Part model, mm, in its own coordinate system. Give positions to 0.01 mm unless a question says otherwise; leave off trailing zeros. Write each loop counter-clockwise with the first axis right and the second up, starting at its lowest first coordinate (ties: lowest second). Pieces come first, ordered by that corner, then holes.
```python
from build123d import *

# Parameters (mm, degrees)
SKETCH1_W               = 279.4
SKETCH1_H               = 90.8685
BOSS_EXTRUDE1_DEPTH     = 2.54
SKETCH2_W               = 12.7
SKETCH2_H               = 2.54
CUT_EXTRUDE1_DEPTH      = 147.92451352
LPATTERN1_COUNT         = 3
LPATTERN1_PITCH         = 25.4
MIRROR1_COPY_1_SKETCH_W = 12.7
MIRROR1_COPY_1_SKETCH_H = 2.54
MIRROR1_COPY_1_DEPTH    = 147.92451352
MIRROR1_COPY_2_SKETCH_W = 12.7
MIRROR1_COPY_2_SKETCH_H = 2.54
MIRROR1_COPY_2_DEPTH    = 147.92451352
SKETCH3_W               = 2.54
SKETCH3_H               = 25.4
CUT_EXTRUDE2_DEPTH      = 147.92451352
LPATTERN2_COUNT         = 2
LPATTERN2_PITCH         = 50.8
MIRROR2_COPY_1_SKETCH_W = 2.54
MIRROR2_COPY_1_SKETCH_H = 25.4
MIRROR2_COPY_1_DEPTH    = 147.92451352
SKETCH4_W               = 2.54
SKETCH4_H               = 12.7
CUT_EXTRUDE3_DEPTH      = 147.92451352
LPATTERN3_COUNT         = 3
LPATTERN3_PITCH         = 25.4
MIRROR3_COPY_1_SKETCH_W = 2.54
MIRROR3_COPY_1_SKETCH_H = 12.7
MIRROR3_COPY_1_DEPTH    = 147.92451352
MIRROR3_COPY_2_SKETCH_W = 2.54
MIRROR3_COPY_2_SKETCH_H = 12.7
MIRROR3_COPY_2_DEPTH    = 147.92451352
SKETCH5_W               = 25.4
SKETCH5_H               = 2.54
SKETCH5_W_2             = 10.76325
CUT_EXTRUDE4_DEPTH      = 147.92451352


with BuildPart() as part:
    # Sketch1 → Boss-Extrude1 (new body)
    with BuildSketch(Plane.XY):
        Rectangle(SKETCH1_W, SKETCH1_H)
    extrude(amount=BOSS_EXTRUDE1_DEPTH)

    # Sketch2 → Cut-Extrude1 (cut, through all)
    with BuildSketch(Plane.XY.offset(2.54)):
        with Locations((139.7, 44.16425)):
            Rectangle(SKETCH2_W, SKETCH2_H)
    cut_extrude1 = extrude(amount=-CUT_EXTRUDE1_DEPTH, mode=Mode.SUBTRACT)

    # LPattern1: Cut-Extrude1 ×3
    with Locations(*[(-i * LPATTERN1_PITCH, 0, 0) for i in range(1, LPATTERN1_COUNT)]):
        add(cut_extrude1, mode=Mode.SUBTRACT)

    # Mirror1: Cut-Extrude1 across plane
    add(cut_extrude1.mirror(Plane(origin=(0, 0, 0), x_dir=(0, 0, 1), z_dir=(1, 0, 0))), mode=Mode.SUBTRACT)

    # Mirror1 copy 1 sketch → Mirror1 copy 1 (cut, through all)
    with BuildSketch(Plane(origin=(25.4, 0, 2.54), x_dir=(-1, 0, 0), z_dir=(0, 0, 1))):
        with Locations((139.7, -44.16425)):
            Rectangle(MIRROR1_COPY_1_SKETCH_W, MIRROR1_COPY_1_SKETCH_H)
    extrude(amount=-MIRROR1_COPY_1_DEPTH, mode=Mode.SUBTRACT)

    # Mirror1 copy 2 sketch → Mirror1 copy 2 (cut, through all)
    with BuildSketch(Plane(origin=(50.8, 0, 2.54), x_dir=(-1, 0, 0), z_dir=(0, 0, 1))):
        with Locations((139.7, -44.16425)):
            Rectangle(MIRROR1_COPY_2_SKETCH_W, MIRROR1_COPY_2_SKETCH_H)
    extrude(amount=-MIRROR1_COPY_2_DEPTH, mode=Mode.SUBTRACT)

    # Sketch3 → Cut-Extrude2 (cut, through all)
    with BuildSketch(Plane.XY.offset(2.54)):
        with Locations((76.327, -38.06825)):
            Rectangle(SKETCH3_W, SKETCH3_H)
    cut_extrude2 = extrude(amount=-CUT_EXTRUDE2_DEPTH, mode=Mode.SUBTRACT)

    # LPattern2: Cut-Extrude2 ×2
    with Locations(*[(0, i * LPATTERN2_PITCH, 0) for i in range(1, LPATTERN2_COUNT)]):
        add(cut_extrude2, mode=Mode.SUBTRACT)

    # Mirror2: Cut-Extrude2 across plane
    add(cut_extrude2.mirror(Plane(origin=(0, 0, 0), x_dir=(0, 0, 1), z_dir=(1, 0, 0))), mode=Mode.SUBTRACT)

    # Mirror2 copy 1 sketch → Mirror2 copy 1 (cut, through all)
    with BuildSketch(Plane(origin=(0, 50.8, 2.54), x_dir=(-1, 0, 0), z_dir=(0, 0, 1))):
        with Locations((76.327, 38.06825)):
            Rectangle(MIRROR2_COPY_1_SKETCH_W, MIRROR2_COPY_1_SKETCH_H)
    extrude(amount=-MIRROR2_COPY_1_DEPTH, mode=Mode.SUBTRACT)

    # Sketch4 → Cut-Extrude3 (cut, through all)
    with BuildSketch(Plane.XY.offset(2.54)):
        with Locations((138.43, -26.38425)):
            Rectangle(SKETCH4_W, SKETCH4_H)
    cut_extrude3 = extrude(amount=-CUT_EXTRUDE3_DEPTH, mode=Mode.SUBTRACT)

    # LPattern3: Cut-Extrude3 ×3
    with Locations(*[(0, i * LPATTERN3_PITCH, 0) for i in range(1, LPATTERN3_COUNT)]):
        add(cut_extrude3, mode=Mode.SUBTRACT)

    # Mirror3: Cut-Extrude3 across plane
    add(cut_extrude3.mirror(Plane(origin=(0, 0, 0), x_dir=(0, 0, 1), z_dir=(1, 0, 0))), mode=Mode.SUBTRACT)

    # Mirror3 copy 1 sketch → Mirror3 copy 1 (cut, through all)
    with BuildSketch(Plane(origin=(0, 25.4, 2.54), x_dir=(-1, 0, 0), z_dir=(0, 0, 1))):
        with Locations((138.43, 26.38425)):
            Rectangle(MIRROR3_COPY_1_SKETCH_W, MIRROR3_COPY_1_SKETCH_H)
    extrude(amount=-MIRROR3_COPY_1_DEPTH, mode=Mode.SUBTRACT)

    # Mirror3 copy 2 sketch → Mirror3 copy 2 (cut, through all)
    with BuildSketch(Plane(origin=(0, 50.8, 2.54), x_dir=(-1, 0, 0), z_dir=(0, 0, 1))):
        with Locations((138.43, 26.38425)):
            Rectangle(MIRROR3_COPY_2_SKETCH_W, MIRROR3_COPY_2_SKETCH_H)
    extrude(amount=-MIRROR3_COPY_2_DEPTH, mode=Mode.SUBTRACT)

    # Sketch5 → Cut-Extrude4 (cut, through all)
    with BuildSketch(Plane.XY.offset(2.54)):
        with Locations((-25.4, 44.16425)):
            Rectangle(SKETCH5_W, SKETCH5_H)
        with Locations((-68.881625, 44.16425)):
            Rectangle(SKETCH5_W_2, SKETCH5_H)
    cut_extrude4 = extrude(amount=-CUT_EXTRUDE4_DEPTH, mode=Mode.SUBTRACT)

    # Mirror4: Cut-Extrude4 across plane
    add(cut_extrude4.mirror(Plane(origin=(0, 0, 0), x_dir=(0, 0, 1), z_dir=(1, 0, 0))), mode=Mode.SUBTRACT)


solid = part.part
```
1) Saw through at C-C, the plane z = 0.65. Count the separate pieces of the cut face and the enclosed holes in it, then the cut area to 3 significant figures.
Answers follow:
separate pieces: 1
enclosed holes: 2
area: 24,600 mm2
2) Saw through at B-B, the plane x = -66.5. Write the cut outline in (y, z).
Answers follow:
outline: (-45.43, 0) - (42.89, 0) - (42.89, 2.54) - (-45.43, 2.54) - close
3) Pin check, flat tip, straight feed: pin 1 Ø1.3 at (y, z) = (44.5, 1.5) entering from +X. Stop position of the tip, or through.
Answers follow:
pin 1: stops at x = 133.35
4) Saw through at A-A, the plane y = 15. Write the cut outline in (x, z), then the cut area to 3 significant figures.
Answers follow:
outline: (-139.7, 0) - (-77.6, 0) - (-77.6, 2.54) - (-139.7, 2.54) - close; (-75.06, 0) - (75.06, 0) - (75.06, 2.54) - (-75.06, 2.54) - close; (77.6, 0) - (139.7, 0) - (139.7, 2.54) - (77.6, 2.54) - close
area: 697 mm2
5) Wall check: L1, parallel to X at y = -32, z = 0.45; L2, parallel to X at y = 18, z = 0.65; L3, parallel to Y at x = 94, z = 1.7. Give the ranges that are in metal, low to high.
Answers follow:
L1: x = -137.16 to -77.6, -75.06 to 75.06, 77.6 to 137.16
L2: x = -139.7 to -77.6, -75.06 to 75.06, 77.6 to 139.7
L3: y = -45.43 to 42.89
